Can you work these out from the model? Positions are in its coordinate system, mm. Coordinates: 2 decimals unless noted, no trailing zeros. Loops run counter-clockwise (first coordinate to the right, second up) from the corner with the lowest first, then second, coordinate; pieces in that order, holes last.
```python
from build123d import *

# Parameters (mm, degrees)
SKETCH_1_W                    = 11.3
SKETCH_1_H                    = 36.3
EXTRUDE_1_DEPTH               = 1.5
CHAMFER_1_SIZE                = 0.4
SKETCH_2_W                    = 1.5
SKETCH_2_H                    = 13
CUT_EXTRUDE_1_DEPTH           = 1
CUT_EXTRUDE_1_DRAFT           = -24
CUT_EXTRUDE_1_PROFILE_2_DEPTH = 1
CUT_EXTRUDE_1_PROFILE_2_DRAFT = -24
CUT_EXTRUDE_2_DEPTH           = 10


with BuildPart() as part:
    # 草图1 → 凸台-拉伸1 (new body)
    with BuildSketch(Plane(origin=(0, 0, 0), x_dir=(1, 0, 0), z_dir=(0, 1, 0))):
        with Locations((5.65, -18.15)):
            Rectangle(SKETCH_1_W, SKETCH_1_H)
    extrude(amount=EXTRUDE_1_DEPTH)

    # 倒角1
    chamfer_1_edges = [part.edges().sort_by_distance(p)[0] for p in [
        (0, 0.75, 0),
        (11.3, 0.75, 0),
        (11.3, 0.75, 36.3),
        (0, 0.75, 36.3),
    ]]
    chamfer(chamfer_1_edges, length=CHAMFER_1_SIZE)


with BuildPart() as cut_extrude_1_tool:
    # 草图2 → 切除-拉伸1 (with draft: the straight prism first)
    with BuildSketch(Plane(origin=(0, 1.5, 0), x_dir=(1, 0, 0), z_dir=(0, 1, 0))):
        with Locations((1.55, -18.15)):
            Rectangle(SKETCH_2_W, SKETCH_2_H)
    extrude(amount=-CUT_EXTRUDE_1_DEPTH)
    # 切除-拉伸1: the draft: its side faces are tilted about the plane it starts from
    cut_extrude_1_sides = [cut_extrude_1_tool.faces().sort_by_distance(p)[0] for p in [
        (0.8, 1, 18.15),
        (1.55, 1, 24.65),
        (2.3, 1, 18.15),
        (1.55, 1, 11.65),
    ]]
    draft(cut_extrude_1_sides, Plane(origin=(0, 1.5, 0), x_dir=(1, 0, 0), z_dir=(0, 1, 0)), CUT_EXTRUDE_1_DRAFT)


with BuildPart() as part_1:
    add(part.part)

    # 切除-拉伸1: cut by cut_extrude_1_tool
    add(cut_extrude_1_tool.part, mode=Mode.SUBTRACT)


with BuildPart() as cut_extrude_1_profile_2_tool:
    # 草图2 → 切除-拉伸1 profile 2 (with draft: the straight prism first)
    with BuildSketch(Plane(origin=(0, 1.5, 0), x_dir=(1, 0, 0), z_dir=(0, 1, 0))):
        with Locations((9.75, -18.15)):
            Rectangle(SKETCH_2_W, SKETCH_2_H)
    extrude(amount=-CUT_EXTRUDE_1_PROFILE_2_DEPTH)
    # 切除-拉伸1 profile 2: the draft: its side faces are tilted about the plane it starts from
    cut_extrude_1_profile_2_sides = [cut_extrude_1_profile_2_tool.faces().sort_by_distance(p)[0] for p in [
        (9.75, 1, 11.65),
        (9, 1, 18.15),
        (9.75, 1, 24.65),
        (10.5, 1, 18.15),
    ]]
    draft(cut_extrude_1_profile_2_sides, Plane(origin=(0, 1.5, 0), x_dir=(1, 0, 0), z_dir=(0, 1, 0)), CUT_EXTRUDE_1_PROFILE_2_DRAFT)


with BuildPart() as part_2:
    add(part_1.part)

    # 切除-拉伸1 profile 2: cut by cut_extrude_1_profile_2_tool
    add(cut_extrude_1_profile_2_tool.part, mode=Mode.SUBTRACT)

    # 草图3 → 切除-拉伸2 (cut)
    with BuildSketch(Plane(origin=(0, 1.5, 0), x_dir=(1, 0, 0), z_dir=(0, 1, 0))):
        Polygon((0, -0.4), (0, -35.9), (0.4, -36.3), (10.9, -36.3), (11.3, -35.9), (11.3, -0.4), (10.9, 0), (0.4, 0), align=None)
        Polygon((0.2, -0.482842712), (0.2, -35.817157288), (0.482842712, -36.1), (10.817157288, -36.1), (11.1, -35.817157288), (11.1, -0.482842712), (10.817157288, -0.2), (0.482842712, -0.2), align=None, mode=Mode.SUBTRACT)
    extrude(amount=-CUT_EXTRUDE_2_DEPTH, mode=Mode.SUBTRACT)


solid = part_2.part
```
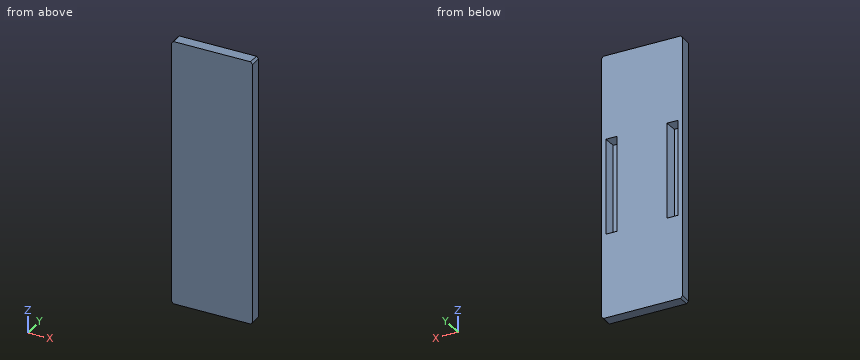
(1) I want a section at C-C on x = 9.75. Write out the boundary of the cut face in (y, z).
Check values:
outline: (0, 0.2) - (1.5, 0.2) - (1.5, 11.65) - (0.5, 12.1) - (0.5, 24.2) - (1.5, 24.65) - (1.5, 36.1) - (0, 36.1) - close
(2) I want a section at A-A on z = 18. Write out the boundary of the cut face in (x, y).
Check values:
outline: (0.2, 0) - (11.1, 0) - (11.1, 1.5) - (10.5, 1.5) - (10.05, 0.5) - (9.45, 0.5) - (9, 1.5) - (2.3, 1.5) - (1.85, 0.5) - (1.25, 0.5) - (0.8, 1.5) - (0.2, 1.5) - close
(3) If I drill on probe 1 along X at (y, z) = (1, 13); probe 2 along X at (y, z) = (0.65, 17); probe 3 along Y at (x, z) = (1.75, 22.5), over which ranges is the centre line in solid material (lowest first)?
Check values:
probe 1: x = 0.2 to 1.02, 2.08 to 9.22, 10.28 to 11.1
probe 2: x = 0.2 to 1.18, 1.92 to 9.38, 10.12 to 11.1
probe 3: y = 0 to 0.5
(4) I want a section at B-B on y = 1.1. Write out the boundary of the cut face in (x, z), then the cut area to 3 significant figures.
Check values:
outline: (0.2, 0.48) - (0.48, 0.2) - (10.82, 0.2) - (11.1, 0.48) - (11.1, 35.82) - (10.82, 36.1) - (0.48, 36.1) - (0.2, 35.82) - close; hole (0.98, 11.83) - (2.12, 11.83) - (2.12, 24.47) - (0.98, 24.47) - close; hole (9.18, 11.83) - (10.32, 11.83) - (10.32, 24.47) - (9.18, 24.47) - close
area: 362 mm2
